Could you check a few things on this model? Use its own coordinates, in mm. Face numbers are marked on the shaded views. A direction names the side the tool comes from. Give positions to 0.01 mm unless a question says otherwise; leave off trailing zeros. Order: outer loops, then holes, each group sorted by start corner. A loop starts at its lowest first (then second) coordinate and runs counter-clockwise, first axis right, second up. Notation, with made-up numbers: M 18.5,49 L 37.5,49 A14 cw 37.5,75 Z; hole C 45.5,-7.75 d1. An arc over 180 degrees is marked long. Use a Markdown table: item, result. Add a question column.
Item 1: Suppose I cut it at B-B on x = -128. Write out the boundary of the cut face in (y, z), plus the area to 3 significant figures.
Item 2: If I drill on L1, parallel to X at y = 159, z = -420; L2, parallel to Z at x = 0, y = 189; L3, parallel to Z at x = -65, y = 137, over which ranges is the centre line in solid material (lowest first)? Write a range as from..to.
Item 3: I'm going to push flat-ended pins straight in: pin 1 Ø3 at (y, z) = (136, -95.5) entering from +X; pin 2 Ø10 at (y, z) = (159.5, 135) entering from -X; pin 3 Ø1 at (y, z) = (329.5, -297) entering from -X. Where does each tip first touch, or does it pass through?
Item 4: Suppose I cut it at D-D on z = 118. Write out the boundary of the cut face in (x, y).
Item 5: If we mould it in two halves opening along X, with no side actions, what happens to the marked faces 4, 5, 6 and 7? For each: released by +X, released by -X, zero draft, split by the parting line, or undercut.
Item 6: Suppose I cut it at C-C on x = 0. Write out the boundary of the cut face in (y, z).
Item 7: Suppose I cut it at A-A on z = -420. Write out the boundary of the cut face in (x, y), plus the area to 3 significant figures.
Item 8: For the marked faces 1, 2 and 3, which set-ups out of +Z, -Z, +X, -X, +Y, -Y let a thin tool reach every point of the face, with its end or its side?
Autodesk Fusion 360 part; units mm, degrees
sketch "Sketch1" plane through (0, 0, 0) normal (0, 1, 0) x (1, 0, 0)
  line L0 (-240, 275.7779) -> (-240, -450)
  line L1 (-240, -450) -> (240, -450)
  line L2 (240, -450) -> (240, 275.7779)
  line L3 (240, 450) -> (-240, -450) construction
  line L4 (-240, 450) -> (240, -450) construction
  line L5 (30, 577.1623) -> (30, 698.3882)
  line L6 (-30, 698.3882) -> (-30, 577.1623)
  arc A0 (-30, 698.3882) -> (30, 698.3882) centre (0, 420) ccw
  arc A1 (-30, 577.1623) -> (30, 577.1623) centre (0, 420) ccw
  dimension "d1" = 480
  dimension "d2" = 900
  dimension "d3" = 560
  dimension "d4" = 420
  dimension "d5" = 320
extrude "Extrude1" add sketch "Sketch1" along normal blind 560 contours L5 L6 A0 A1 makes body 1
extrude "Extrude2" add sketch "Sketch1" along normal blind 240 separate body contours L0 L1 L2 A0 makes body 2
sketch "Sketch2" plane through (0, 0, 450) normal (0, 0, 1) x (1, 0, 0)
  line L0 (-240, 0) -> (240, 0)
  line L1 (240, 0) -> (240, 240)
  line L2 (240, 240) -> (-240, 240)
  line L3 (-240, 240) -> (-240, 0)
  circle A0 centre (0, 240) radius 80
  dimension "d12" = 160
extrude "Extrude3" cut sketch "Sketch2" against normal blind 400 contours L2 A0 picked at (-9.7424, 215.1767) bodies 2
combine "Combine1" operation add target body 1 tool bodies 2
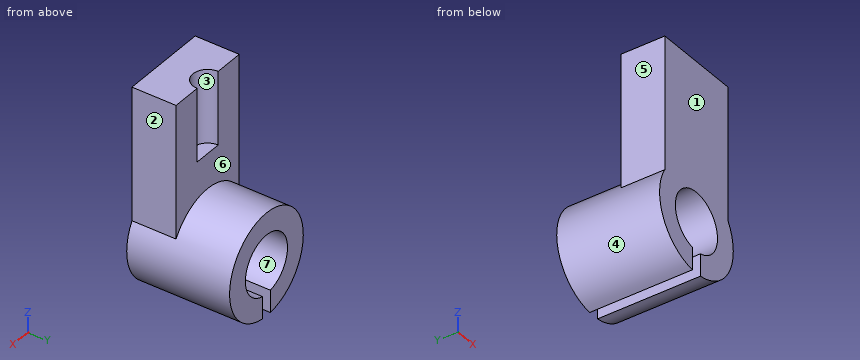
Findings below:
| question | item | result |
|---|---|---|
| 1 | outline | M 0,-669.03 L 560,-669.03 L 560,-516 L 0,-516 Z; M 0,-324 L 560,-324 L 560,-170.97 L 240,-170.97 L 240,450 L 0,450 Z |
| 1 | area | 320,000 mm^2 |
| 2 | L1 | x = -280..-160, 160..280 |
| 2 | L2 | z = -260..50 |
| 2 | L3 | z = -692.35..-566.2, -273.8..450 |
| 3 | pin 1 | stops at x = 240 |
| 3 | pin 2 | stops at x = -240 |
| 3 | pin 3 | stops at x = -251.78 |
| 4 | outline | M -240,0 L 240,0 L 240,240 L 80,240 A80 cw -80,240 L -240,240 Z |
| 5 | face 4 | split by the parting line |
| 5 | face 5 | released by -X |
| 5 | face 6 | zero draft |
| 5 | face 7 | undercut |
| 6 | outline | M 0,-260 L 560,-260 L 560,-140 L 240,-140 L 240,50 L 160,50 L 160,450 L 0,450 Z |
| 7 | outline | M -280,0 L -160,0 L -160,560 L -280,560 Z; M 160,0 L 280,0 L 280,560 L 160,560 Z |
| 7 | area | 134,000 mm^2 |
| 8 | face 1 | +Z, -Z, +X, -X, -Y |
| 8 | face 2 | +Z, +X, +Y, -Y |
| 8 | face 3 | +Z, +Y |
